Check sheet for the modelled part. Datum: model origin and axes. Units: mm. A direction names the side the tool comes from. Coordinates: 2 decimals unless noted, no trailing zeros. Loops run counter-clockwise (first coordinate to the right, second up) from the corner with the lowest first, then second, coordinate; pieces in that order, holes last.
from build123d import *

# Parameters (mm, degrees)
SKETCH1_R           = 50
SKETCH1_W           = 100
SKETCH1_H           = 100
SKETCH1_H_2         = 160
BOSS_EXTRUDE1_DEPTH = 50


with BuildPart() as part:
    # Sketch1 → Boss-Extrude1 (new body)
    with BuildSketch(Plane(origin=(0, 0, 0), x_dir=(1, 0, 0), z_dir=(0, 1, 0))):
        with BuildLine():
            Line((-157.631299989, 88.07121729), (-136.663415109, 133.755017511))
            Line((-136.663415109, 133.755017511), (-135.958224263, 135.291452776))
            ThreePointArc((-135.958224263, 135.291452776), (-127.47369707, 169.829345008), (-132.36344953, 205.056373302))
            ThreePointArc((-132.36344953, 205.056373302), (0, 389.785594222), (132.36344953, 205.056373302))
            ThreePointArc((132.36344953, 205.056373302), (127.47369707, 169.829345008), (135.958224263, 135.291452776))
            Line((135.958224263, 135.291452776), (136.663415109, 133.755017511))
            Line((136.663415109, 133.755017511), (157.631299989, 88.07121729))
            ThreePointArc((157.631299989, 88.07121729), (178.287067415, 59.119663384), (208.18524924, 39.859551103))
            ThreePointArc((208.18524924, 39.859551103), (275.706725604, -162.3983111), (65.252859665, -196.699373836))
            ThreePointArc((65.252859665, -196.699373836), (44.010636723, -184.306940013), (19.797939242, -180))
            Line((19.797939242, -180), (-19.797939242, -180))
            ThreePointArc((-19.797939242, -180), (-44.010636723, -184.306940013), (-65.252859665, -196.699373836))
            ThreePointArc((-65.252859665, -196.699373836), (-275.706725604, -162.3983111), (-208.18524924, 39.859551103))
            ThreePointArc((-208.18524924, 39.859551103), (-178.287067415, 59.119663384), (-157.631299989, 88.07121729))
        make_face()
        with Locations(Location((0, 250, 0), (0, 0, 270))):
            Circle(SKETCH1_R, mode=Mode.SUBTRACT)
        Rectangle(SKETCH1_W, SKETCH1_H, mode=Mode.SUBTRACT)
        with Locations((155.884572681, -90)):
            Rectangle(SKETCH1_W, SKETCH1_H_2, mode=Mode.SUBTRACT)
        with Locations((-155.884572681, -90)):
            Rectangle(SKETCH1_W, SKETCH1_H_2, mode=Mode.SUBTRACT)
    extrude(amount=BOSS_EXTRUDE1_DEPTH)


solid = part.part
(1) Section check C-C, the plane z = 90. Enter the section's corners in (x, y).
(2) Section check A-A, the plane z = -250. Enter the section's corners in (x, y), plus the area to 3 significant figures.
(3) Gauge pin test, flat ends, axial feed: P1, Ø12, axis at x = 151, y = 30, coming from the -Z side; P2, Ø15, axis at y = 18.5, z = 103, coming from the +X side; P3, Ø25, axis at x = 160, y = 25, coming from the -Z side. Record the tip position at first contact, or that the pin passes through.
(4) Set-up check for faces 1 (the face through (105.885, 25, 91)), 2 (the face through (44.34, 24.65, 184.43)), 3 (the face through (177.926, 24.65, -59.466)): record each of +Z, -Z, +X, -X, +Y, -Y from which the full face is reachable in a straight line by a thin tool's end or side.
(5) Section check B-B, the plane x = 0. Enter the section's corners in (y, z), plus the area to 3 significant figures.
(6) Scan lines: line 1 along X through (y, z) = (13.5, -250); line 2 along Z through (x, y) = (31, 18); line 3 along X through (y, z) = (22.5, -177). Record each from-to range of solid material in increasing order.
(7) Draft check along Z on faces 4 (the face through (-273.917, 24.65, 165.281)), 5 (the face through (127.45, 24.65, -170.33)), 6 (the face through (4, 50, -84)). Enter one of: pulls with the +Z half, pulls with the -Z half, needs draft (parallel to the pull), parting line crosses it, or undercut.
(8) Section check D-D, the plane y = 22. Enter the section's corners in (x, z), plus the area to 3 significant figures.
Determined:
1. outline: (-295.88, 0) - (-205.88, 0) - (-205.88, 50) - (-295.88, 50) - close; (-105.88, 0) - (105.88, 0) - (105.88, 50) - (-105.88, 50) - close; (205.88, 0) - (295.88, 0) - (295.88, 50) - (205.88, 50) - close
2. outline: (-139.79, 0) - (-50, 0) - (-50, 50) - (-139.79, 50) - close; (50, 0) - (139.79, 0) - (139.79, 50) - (50, 50) - close
2. area: 8,980 mm2
3. P1: stops at z = -115.59
3. P2: stops at x = 295.77
3. P3: stops at z = -110.14
4. face 1: +Y, -Y
4. face 2: +Z, +Y, -Y
4. face 3: -Z, +X, +Y, -Y
5. outline: (0, -389.79) - (50, -389.79) - (50, -300) - (0, -300) - close; (0, -200) - (50, -200) - (50, -50) - (0, -50) - close; (0, 50) - (50, 50) - (50, 180) - (0, 180) - close
5. area: 18,500 mm2
6. line 1: x = -139.79 to -50, 50 to 139.79
6. line 2: z = -386.3 to -289.23, -210.77 to -50, 50 to 180.9
6. line 3: x = -127.38 to 127.38
7. face 4: parting line crosses it
7. face 5: undercut
7. face 6: needs draft
8. outline: (-208.19, -39.86) arc R94.45 cw to (-157.63, -88.07) - (-135.96, -135.29) arc R94.45 cw to (-132.36, -205.06) arc R139.79 ccw (long way) to (132.36, -205.06) arc R94.45 cw to (135.96, -135.29) - (157.63, -88.07) arc R94.45 cw to (208.19, -39.86) arc R140 ccw (long way) to (65.25, 196.7) arc R70.21 cw to (19.8, 180) - (-19.8, 180) arc R70.21 cw to (-65.25, 196.7) arc R140 ccw (long way) to start; hole (-205.88, 10) - (-105.88, 10) - (-105.88, 170) - (-205.88, 170) - close; hole circle Ø100 at (0, -250); hole (-50, -50) - (50, -50) - (50, 50) - (-50, 50) - close; hole (105.88, 10) - (205.88, 10) - (205.88, 170) - (105.88, 170) - close
8. area: 179,000 mm2
